Geometry check sheet. Reference: drawing and pictorial views, mm from the part's lowest x, y, z. A direction names the side the tool comes from. Give positions to 0.01 mm unless a question says otherwise; leave off trailing zeros. Order: outer loops, then holes, each group sorted by start corner. A loop starts at its lowest first (then second) coordinate and runs counter-clockwise, first axis right, second up. Notation, with made-up numbers: M -6.5,8 L 6.5,8 A13 cw 6.5,24 Z; hole C 10.5,-31.5 d10. An arc over 180 degrees is marked long. Answer as CSV lines item,"result".
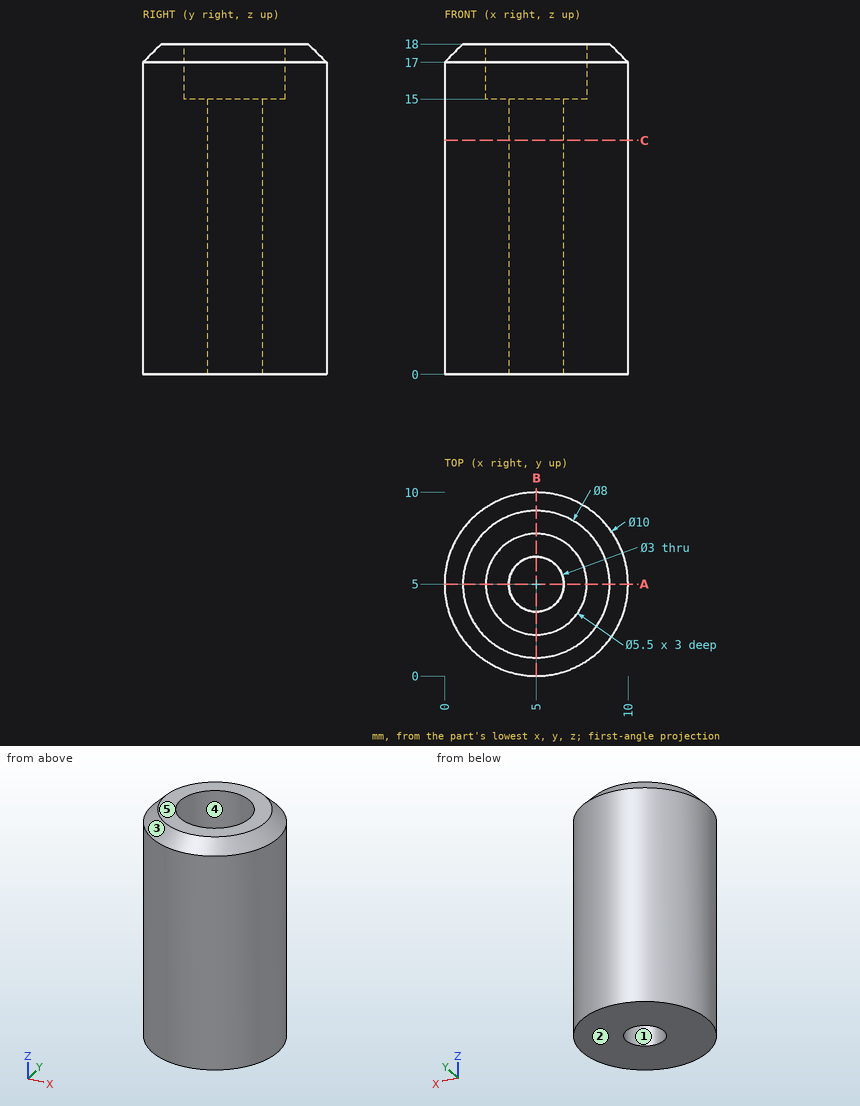
(1) Gauge pin test, flat end, axial feed: P1, Ø1, axis at x = 3, y = 5, coming from the +Z side. Record the tip position at first contact, or that the pin passes through.
The answers:
P1,"stops at z = 15"
(2) Material ranges on line 1 (Y direction, x = 5, z = 10.5); line 2 (Y direction, x = 5, z = 16.2); line 3 (Z direction, x = 2.75, y = 5.5), recorded low to high.
The answers:
line 1,"y = 0 to 3.5, 6.5 to 10"
line 2,"y = 0 to 2.25, 7.75 to 10"
line 3,"z = 0 to 15"
(3) Draft check along Y on the marked faces 1, 2 and 3. Enter one of: +Y half, -Y half, draft (parallel to the pull), parting line (faces both ways), or undercut.
The answers:
face 1,"undercut"
face 2,"draft"
face 3,"parting line"
(4) Section check A-A on y = 5. Enter the section's corners in (x, z).
The answers:
outline,"M 0,0 L 3.5,0 L 3.5,15 L 2.25,15 L 2.25,18 L 1,18 L 0,17 Z; M 6.5,0 L 10,0 L 10,17 L 9,18 L 7.75,18 L 7.75,15 L 6.5,15 Z"
(5) Tool access check on the marked faces 4 and 5. Record the directions out of +Z, -Z, +X, -X, +Y, -Y that give a thin tool (end or side, any length) a straight path to the whole face; none if there is none.
The answers:
face 4,"+Z"
face 5,"+Z, +X, -X, +Y, -Y"
(6) Section check C-C on z = 12.75. Enter the section's corners in (x, y).
The answers:
outline,"C 5,5 d10; hole C 5,5 d3"
